```python
from build123d import *

# Parameters (mm, degrees)
BOSS_EXTRUDE2_DEPTH = 9
SKETCH2_W           = 9
SKETCH2_H           = 9
CUT_EXTRUDE1_DEPTH  = 126.837196409
BOSS_EXTRUDE3_DEPTH = 9


with BuildPart() as part:
    # Sketch1 → Boss-Extrude2 (new body)
    with BuildSketch(Plane.XY):
        with BuildLine():
            Line((-123, 25), (-123, 0))
            Line((-123, 0), (123, 0))
            Line((123, 0), (123, 25))
            Line((123, 25), (114, 25))
            ThreePointArc((114, 25), (0, 12.5), (-114, 25))
            Line((-114, 25), (-123, 25))
        make_face()
    extrude(amount=BOSS_EXTRUDE2_DEPTH)

    # Sketch2 → Cut-Extrude1 (cut, through all)
    with BuildSketch(Plane.XY):
        with Locations((118.5, 13.5)):
            Rectangle(SKETCH2_W, SKETCH2_H)
        with Locations((-118.5, 13.5)):
            Rectangle(SKETCH2_W, SKETCH2_H)
    extrude(amount=CUT_EXTRUDE1_DEPTH, mode=Mode.SUBTRACT)

    # Sketch3 → Boss-Extrude3 (add)
    with BuildSketch(Plane.XY):
        Polygon((114, 25), (114, 0), (150, 0), (150, 9), (141, 9), (141, 18), (150, 18), (150, 25), align=None)
    extrude(amount=BOSS_EXTRUDE3_DEPTH)


solid = part.part
```
The model under review builds one solid part; all positions refer to its coordinate system, in mm. A direction names the side the tool comes from. Coordinates: 2 decimals unless noted, no trailing zeros. Order: outer loops, then holes, each group sorted by start corner. A loop starts at its lowest first (then second) coordinate and runs counter-clockwise, first axis right, second up. Notation, with made-up numbers: (42, -27.5) -> (50, -27.5) arc R9 ccw to (50, -17.5) -> close; hole circle Ø1 at (-31.5, 64). An arc over 180 degrees is marked (long way). Answer in a Markdown table with one row per item. Add a question column.
Item 1: We need section D-D on x = 29. Write out the cut boundary in (y, z), plus the area to 3 significant figures.
Item 2: We need section B-B on z = 1.5. Write out the cut boundary in (x, y), plus the area to 3 significant figures.
Item 3: To check wall thickness, follow probe 1 along X at (y, z) = (11.5, 8.25); probe 2 along Y at (x, z) = (96.5, 7); probe 3 along Y at (x, z) = (61, 7). State the ranges of each line that lie inside material, in increasing order.
Item 4: We need section C-C on x = -55. Write out the cut boundary in (y, z), plus the area to 3 significant figures.
Item 5: Clearance check with a flat-ended pin moving along its axis: pin 1 (2 mm diameter, centred on y = 11.5, z = 1.5, fed in from -X). State where the tip first meets the part, or that it passes through.
Item 6: We need section A-A on y = 20.75. Write out the cut boundary in (x, z), plus the area to 3 significant figures.
Item 7: Machinability: for faces 1 (the flat face through (-119, 18, 4)), 2 (the flat face through (145, 18, 4)), 3 (the flat face through (12, 0, 4)), which of the approach directions +Z, -Z, +X, -X, +Y, -Y give a long, thin tool a straight path to every point of the face, cutting with its end or side? Answer none if there is none.
Final values:
| question | item | result |
|---|---|---|
| 1 | outline | (0, 0) -> (13.3, 0) -> (13.3, 9) -> (0, 9) -> close |
| 1 | area | 120 mm2 |
| 2 | outline | (-123, 0) -> (150, 0) -> (150, 9) -> (141, 9) -> (141, 18) -> (150, 18) -> (150, 25) -> (114, 25) arc R526.09 cw to (-114, 25) -> (-123, 25) -> (-123, 18) -> (-114, 18) -> (-114, 9) -> (-123, 9) -> close |
| 2 | area | 4,760 mm2 |
| 3 | probe 1 | x = -114 to 141 |
| 3 | probe 2 | y = 0 to 21.43 |
| 3 | probe 3 | y = 0 to 16.05 |
| 4 | outline | (0, 0) -> (15.38, 0) -> (15.38, 9) -> (0, 9) -> close |
| 4 | area | 138 mm2 |
| 5 | pin 1 | stops at x = -114 |
| 6 | outline | (-123, 0) -> (-92.8, 0) -> (-92.8, 9) -> (-123, 9) -> close; (92.8, 0) -> (150, 0) -> (150, 9) -> (92.8, 9) -> close |
| 6 | area | 787 mm2 |
| 7 | face 1 | +Z, -Z, -X |
| 7 | face 2 | +Z, -Z, +X |
| 7 | face 3 | +Z, -Z, +X, -X, -Y |
